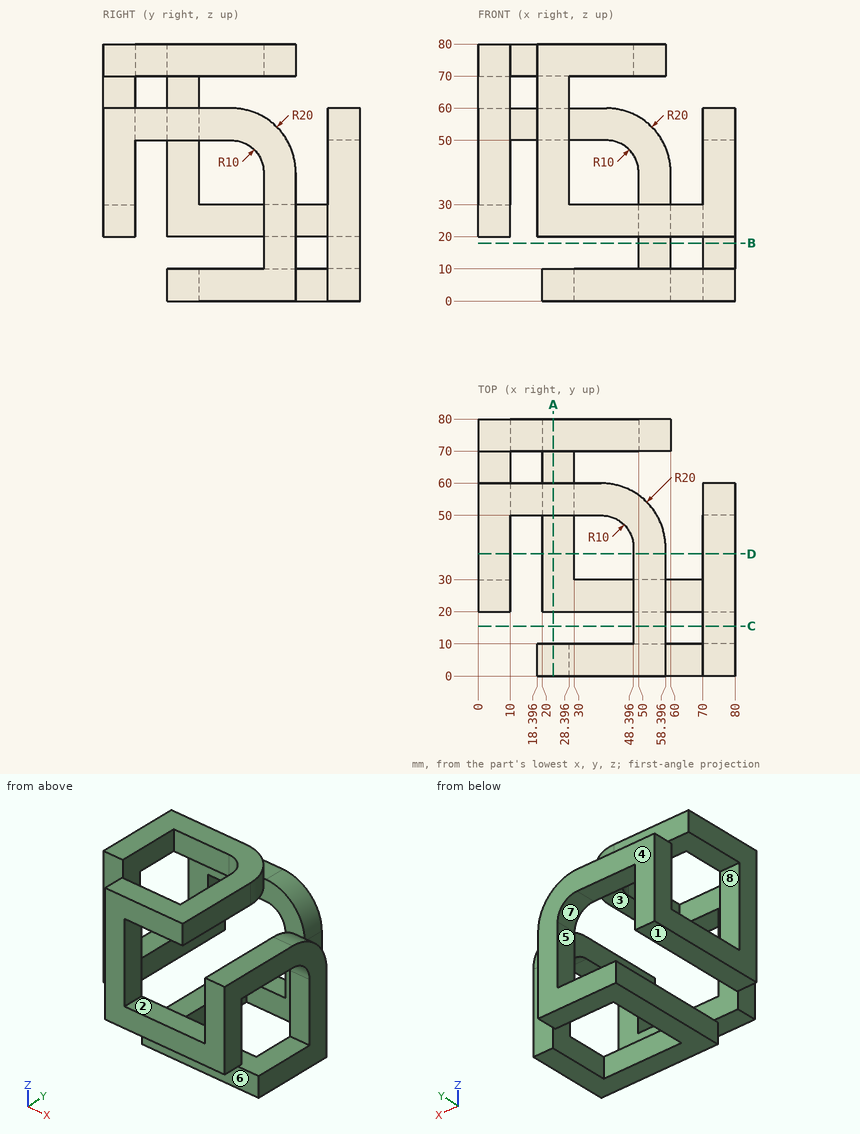
Source: three-view drawing plus pictorial views. Frame: mm from the lowest corner of the part. A direction names the side the tool comes from. Round coordinates to 2 decimals unless told otherwise and drop trailing zeros. Loops run counter-clockwise (first coordinate to the right, second up) from the corner with the lowest first, then second, coordinate; pieces in that order, holes last.
1. Section query D-D on y = 38. Output: boundary loops of the cut face in (x, z).
2. Section query B-B on z = 18. Output: boundary loops of the cut face in (x, y), and give its area (3 significant figures).
3. Access query for the marked faces 5, 6, 7 and 8. Directions: +Z, -Z, +X, -X, +Y, -Y. A direction counts if a zero-diameter tool reaches every point of the face in a straight line with its end or side. Return the directions, or none.
4. Section query C-C on y = 15.5. Output: boundary loops of the cut face in (x, z).
5. Ray query, L1, parallel to X at y = 25, z = 70.5; L2, parallel to Z at x = 28, y = 74.5. Return the intervals inside material, ascending.
6. Contact query for flat-ended pins moving along their axis: pin 1 (8 mm diameter, centred on x = 68.5, z = 43, fed in from +Y); pin 2 (11 mm diameter, centred on y = 42, z = 5.5, fed in from -X); pin 3 (8 mm diameter, centred on y = 25.5, z = 69.5, fed in from -X); pin 4 (3 mm diameter, centred on x = 26, y = 38.5, fed in from +Z). Output: stop coordinate, or through.
7. Section query A-A on x = 23.5. Output: boundary loops of the cut face in (y, z).
8. Mould query, pull axis Z, two halves, no side actions, for the marked faces 1, 2, 3 and 4. Classes: released by +Z, released by -Z, zero draft, split by the parting line, or undercut.
Answers below:
1. outline: (0, 20) - (10, 20) - (10, 30) - (0, 30) - close; (0, 70) - (10, 70) - (10, 80) - (0, 80) - close; (20, 0) - (30, 0) - (30, 10) - (20, 10) - close; (48.4, 70) - (58.4, 70) - (58.4, 80) - (48.4, 80) - close; (70, 0) - (80, 0) - (80, 10) - (70, 10) - close; (70, 50) - (80, 50) - (80, 60) - (70, 60) - close
2. outline: (50, 70) - (60, 70) - (60, 80) - (50, 80) - close; (70, 50) - (80, 50) - (80, 60) - (70, 60) - close
2. area: 200 mm2
3. face 5: +Y
3. face 6: -Z, +X, -X, -Y
3. face 7: +Y, -Y
3. face 8: -X
4. outline: (48.4, 70) - (58.4, 70) - (58.4, 80) - (48.4, 80) - close; (70, 50) - (80, 50) - (80, 60) - (70, 60) - close
5. L1: x = 0 to 10, 48.4 to 58.4
5. L2: z = 0 to 10, 50 to 60
6. pin 1: stops at y = 60
6. pin 2: stops at x = 20
6. pin 3: stops at x = 0
6. pin 4: stops at z = 10
7. outline: (0, 20) - (10, 20) - (10, 80) - (0, 80) - close; (20, 0) - (80, 0) - (80, 10) - (20, 10) - close; (50, 70) - (60, 70) - (60, 80) - (50, 80) - close; (70, 50) - (80, 50) - (80, 60) - (70, 60) - close
8. face 1: released by -Z
8. face 2: undercut
8. face 3: undercut
8. face 4: zero draft
